Model file for the job. Use its own axes, mm. Face numbers are marked on the shaded views. Give positions to 0.01 mm unless a question says otherwise; leave off trailing zeros. Loops run counter-clockwise (first coordinate to the right, second up) from the corner with the lowest first, then second, coordinate; pieces in that order, holes last. Notation, with made-up numbers: (82, 85.25) - (100, 85.25) arc R22 ccw to (100, 119.25) - close; hole circle Ø10 at (4, -14.5). An arc over 180 degrees is marked (long way). Use a Markdown table: item, result.
from build123d import *

# Parameters (mm, degrees)
F0_W      = 65
F0_H      = 215
F1_DEPTH  = 10
F2_SIZE   = 20
F4_DEPTH  = 40
F6_DEPTH  = 10
F7_SIZE   = 6
F9_D      = 30
F10_D     = 24
F12_DEPTH = 60.001
F13_R     = 6
F14_DEPTH = 10
F17_D     = 5
F17_DEPTH = 27.6629407771


with BuildPart() as f1:
    # F0 (on Front) → F1 (new body)
    with BuildSketch(Plane.XZ):
        Rectangle(F0_W, F0_H)
    extrude(amount=-F1_DEPTH)

    # F2
    f2_edges = [f1.edges().sort_by_distance(p)[0] for p in [
        (-32.5, 5, 107.5),
        (32.5, 5, 107.5),
    ]]
    chamfer(f2_edges, length=F2_SIZE)

    # F3 (on face) → F4 (join)
    with BuildSketch(Plane(origin=(0, 10, 0), x_dir=(-1, 0, 0), z_dir=(0, 1, 0))):
        with BuildLine():
            ThreePointArc((8.49e-08, -107.5), (22.9809704186, -97.9809703586), (32.5, -75))
            ThreePointArc((32.5, -75), (0, -42.5), (-32.5, -75))
            ThreePointArc((-32.5, -75), (-22.9809703586, -97.9809704186), (8.49e-08, -107.5))
        make_face()
    extrude(amount=F4_DEPTH)

    # F5 (on face) → F6 (join)
    with BuildSketch(Plane(origin=(0, 50, 0), x_dir=(-1, 0, 0), z_dir=(0, 1, 0))):
        with BuildLine():
            ThreePointArc((-32.5, -75), (0, -42.5), (32.5, -75))
            Line((32.5, -75), (32.5, 57.5))
            Line((32.5, 57.5), (-32.5, 57.5))
            Line((-32.5, 57.5), (-32.5, -75))
        make_face()
        with BuildLine():
            ThreePointArc((-32.5, -75), (-22.9809704241, -97.980970353), (-1.006e-07, -107.5))
            ThreePointArc((-1.006e-07, -107.5), (22.980970353, -97.9809704241), (32.5, -75))
            ThreePointArc((32.5, -75), (0, -42.5), (-32.5, -75))
        make_face()
        with BuildLine():
            Line((-32.5, -107.5), (-1.006e-07, -107.5))
            ThreePointArc((-1.006e-07, -107.5), (-22.9809704241, -97.980970353), (-32.5, -75))
            Line((-32.5, -75), (-32.5, -107.5))
        make_face()
        with BuildLine():
            Line((-1.006e-07, -107.5), (32.5, -107.5))
            Line((32.5, -107.5), (32.5, -75))
            ThreePointArc((32.5, -75), (22.980970353, -97.9809704241), (-1.006e-07, -107.5))
        make_face()
    extrude(amount=F6_DEPTH)

    # F7
    f7_edges = [f1.edges().sort_by_distance(p)[0] for p in [
        (32.5, 55, 57.5),
        (-32.5, 55, 57.5),
    ]]
    chamfer(f7_edges, length=F7_SIZE)

    # F9 (through all)
    with Locations(Plane.XZ):
        with Locations((0, -75)):
            Hole(F9_D / 2)

    # F10 (through all)
    with Locations(Plane.XZ):
        with Locations((0, 32.5)):
            Hole(F10_D / 2)

    # F11 (on face) → F12 (cut, through all)
    with BuildSketch(Plane.XZ):
        with BuildLine():
            ThreePointArc((-6.4644660941, -88.5355339059), (-10.6066017178, -85.6066017178), (-13.5355339059, -81.4644660941))
            Line((-13.5355339059, -81.4644660941), (-16.4755880016, -84.4045201898))
            Line((-16.4755880016, -84.4045201898), (-9.4045201898, -91.4755880016))
            Line((-9.4045201898, -91.4755880016), (-6.4644660941, -88.5355339059))
        make_face()
    extrude(amount=-F12_DEPTH, mode=Mode.SUBTRACT)

    # F13 (on face) → F14 (cut, through all)
    with BuildSketch(Plane.XZ):
        with Locations((0, 93.5)):
            Circle(F13_R)
    extrude(amount=-F14_DEPTH, mode=Mode.SUBTRACT)

    # F17 (through all, one way)
    with BuildSketch(Plane(origin=(-50.4400540957, 0, -50.4400540957), x_dir=(0, -1, 0), z_dir=(0.7071067812, 0, 0.7071067812))):
        with Locations((-30, 53.033008589)):
            Circle(F17_D / 2)
    extrude(amount=-F17_DEPTH, mode=Mode.SUBTRACT)


solid = f1.part
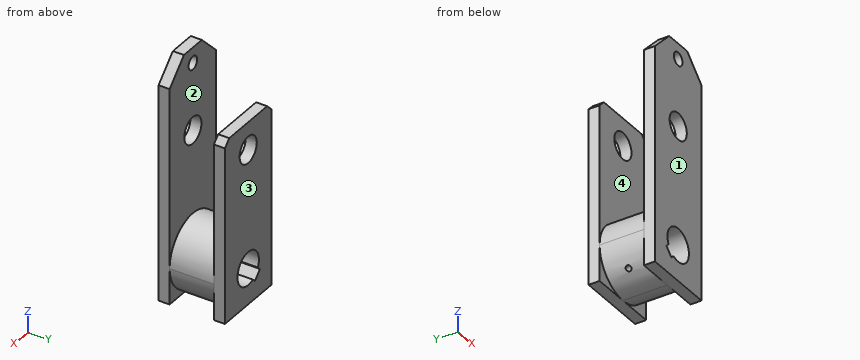
(1) Slice it at B-B, the plane z = 32.5. Write the cut outline in (x, y).
Computed:
| item | result |
|---|---|
| outline | (-32.5, 0) - (-12, 0) - (-12, 10) - (-32.5, 10) - close; (-32.5, 50) - (-12, 50) - (-12, 60) - (-32.5, 60) - close; (12, 0) - (32.5, 0) - (32.5, 10) - (12, 10) - close; (12, 50) - (32.5, 50) - (32.5, 60) - (12, 60) - close |
(2) Slice it at C-C, the plane y = 36.5. Write the cut outline in (x, z).
Computed:
| item | result |
|---|---|
| outline | circle Ø65 at (0, -75); hole (-16.48, -84.4) - (-9.4, -91.48) - (-6.46, -88.54) arc R15 ccw (long way) to (-13.54, -81.46) - close |
(3) Mould opens along Y. For the marked faces 1, 2, 3 and 4 say: pulls with the +Y half, pulls with the -Y half, needs draft (parallel to the pull), parting line crosses it, or undercut.
Computed:
| item | result |
|---|---|
| face 1 | pulls with the -Y half |
| face 2 | undercut |
| face 3 | pulls with the +Y half |
| face 4 | undercut |
(4) Slice it at D-D, the plane x = 4. Write the cut outline in (y, z).
Computed:
| item | result |
|---|---|
| outline | (0, -107.5) - (10, -107.5) - (10, -107.25) - (50, -107.25) - (50, -107.5) - (60, -107.5) - (60, -89.46) - (0, -89.46) - close; (0, -60.54) - (60, -60.54) - (60, 21.19) - (50, 21.19) - (50, -42.75) - (10, -42.75) - (10, 21.19) - (0, 21.19) - close; (0, 43.81) - (10, 43.81) - (10, 89.03) - (0, 89.03) - close; (0, 97.97) - (10, 97.97) - (10, 107.5) - (0, 107.5) - close; (50, 43.81) - (60, 43.81) - (60, 57.5) - (50, 57.5) - close |
(5) Slice it at A-A, the plane z = 93.5. Write the cut outline in (x, y), plus the area to 3 significant figures.
Computed:
| item | result |
|---|---|
| outline | (-26.5, 0) - (-6, 0) - (-6, 10) - (-26.5, 10) - close; (6, 0) - (26.5, 0) - (26.5, 10) - (6, 10) - close |
| area | 410 mm² |
(6) Pin check, flat tips, straight feed: P1, Ø2, axis at x = -16.5, y = 25, coming from the +Z side; P2, Ø1, axis at y = 33, z = -84, coming from the +X side; P3, Ø10, axis at x = -24, y = 31.5, coming from the -Z side; P4, Ø9.5, axis at x = 0, z = 93.5, coming from the +Y side. Stop position of each tip, or through.
Computed:
| item | result |
|---|---|
| P1 | z = -46.43 |
| P2 | x = 31.37 |
| P3 | z = -101.37 |
| P4 | through |
(7) Drill centre lines: probe 1 along Z at (x, y) = (0, 53.5); probe 2 along Z at (x, y) = (-2, 55.5); probe 3 along X at (y, z) = (24, -75). Where is each one in solid material? Low to high. Write a range as [from, to].
Computed:
| item | result |
|---|---|
| probe 1 | [-107.5, -90], [-60, 20.5], [44.5, 57.5] |
| probe 2 | [-107.5, -89.87], [-60.13, 20.67], [44.33, 57.5] |
| probe 3 | [-32.5, -15], [15, 32.5] |
